```python
from build123d import *

# Parameters (mm, degrees)
F0_W     = 12.7
F0_H     = 1.27
F1_DEPTH = 12.7
F2_R     = 5.08


with BuildPart() as f1:
    # F0 (on Right) → F1 (new body, symmetric)
    with BuildSketch(Plane.YZ):
        with Locations((9.525, 50.165)):
            Rectangle(F0_W, F0_H)
        Polygon((3.175, -50.8), (3.175, 49.53), (3.175, 50.8), (-3.175, 50.8), (-3.175, -50.8), (-3.153914, -50.8), align=None)
        Polygon((15.875, -50.8), (22.225, -50.8), (22.225, 50.8), (15.875, 50.8), (15.875, 49.53), align=None)
        with BuildLine():
            Line((3.175, -57.128914), (3.175, -50.8))
            Line((3.175, -50.8), (-3.153914, -50.8))
            ThreePointArc((-3.153914, -50.8), (-1.300218, -55.275218), (3.175, -57.128914))
        make_face()
    extrude(amount=F1_DEPTH, both=True)

    # F2
    f2_edges = [f1.edges().sort_by_distance(p)[0] for p in [
        (0, 22.225, 50.8),
        (0, -3.175, 50.8),
        (0, 22.225, -50.8),
    ]]
    fillet(f2_edges, radius=F2_R)


solid = f1.part
```
The model under review builds one solid part; all positions refer to its coordinate system, in mm. A direction names the side the tool comes from. Round coordinates to 2 decimals unless told otherwise and drop trailing zeros. Order: outer loops, then holes, each group sorted by start corner. A loop starts at its lowest first (then second) coordinate and runs counter-clockwise, first axis right, second up.
Item 1: Add section D-D, the plane y = -1. State the section outline as (x, z) points.
Working result:
outline: (-12.7, -55.56) - (12.7, -55.56) - (12.7, 49.89) - (-12.7, 49.89) - close
Item 2: Add section C-C, the plane y = 6.75. State the section outline as (x, z) points, and give its area (3 significant figures).
Working result:
outline: (-12.7, 49.53) - (12.7, 49.53) - (12.7, 50.8) - (-12.7, 50.8) - close
area: 32.3 mm2
Item 3: Add section A-A, the plane z = 28. State the section outline as (x, y) points (3 decimals).
Working result:
outline: (-12.7, -3.175) - (12.7, -3.175) - (12.7, 3.175) - (-12.7, 3.175) - close; (-12.7, 15.875) - (12.7, 15.875) - (12.7, 22.225) - (-12.7, 22.225) - close
Item 4: Machinability: for faces 1 (the flat face through (0, 3.175, -5)), 2 (the cylindrical face through (0.178, -1.349, -55.226)), which of the approach directions +Z, -Z, +X, -X, +Y, -Y give a long, thin tool a straight path to every point of the face, cutting with its end or side? Answer none if there is none.
Working result:
face 1: -Z, +X, -X
face 2: -Z, +X, -X, -Y
Item 5: To check wall thickness, follow probe 1 along Y at (x, z) = (-1.5, 16) (3 decimals); probe 2 along Z at (x, y) = (-1.5, 8.25); probe 3 along Z at (x, y) = (6.5, 1.25). State the ranges of each line that lie inside material, in increasing order.
Working result:
probe 1: y = -3.175 to 3.175, 15.875 to 22.225
probe 2: z = 49.53 to 50.8
probe 3: z = -56.83 to 50.76
Item 6: For pin 1 (6 mm diameter, centred on x = -1.5, y = 0.5, fed in from -Z); pin 2 (2 mm diameter, centred on x = 6, y = 5, fed in from -Z); pin 3 (2 mm diameter, centred on x = -6, y = 18, fed in from -Z), all flat-tipped, find the tip position at first contact; note any pin that passes through.
Working result:
pin 1: stops at z = -57.13
pin 2: stops at z = 49.53
pin 3: stops at z = -50.8
Item 7: Add section B-B, the plane x = 6. State the section outline as (y, z) points (3 decimals).
Working result:
outline: (-3.175, -50.8) - (-3.154, -50.8) arc R6.329 ccw to (3.175, -57.129) - (3.175, 49.53) - (15.875, 49.53) - (15.875, -50.8) - (17.145, -50.8) arc R5.08 ccw to (22.225, -45.72) - (22.225, 45.72) arc R5.08 ccw to (17.145, 50.8) - (1.905, 50.8) arc R5.08 ccw to (-3.175, 45.72) - close
Item 8: Draft analysis for pull direction Y (two halves, no side actions). For faces 3 (the flat face through (0, -3.175, -2)), 4 (the flat face through (12.7, 1, -2)), 5 (the flat face through (0, 15.875, 0)), state which applies: released by +Y, released by -Y, zero draft, split by the parting line, or undercut.
Working result:
face 3: released by -Y
face 4: zero draft
face 5: undercut
